Part model, mm, in its own coordinate system. Face numbers are marked on the shaded views. A direction names the side the tool comes from. Round coordinates to 2 decimals unless told otherwise and drop trailing zeros. Loops run counter-clockwise (first coordinate to the right, second up) from the corner with the lowest first, then second, coordinate; pieces in that order, holes last. Notation, with made-up numbers: M -5.5,7 L 52.5,7 A38 cw 52.5,46 Z; hole C 2.5,-27 d1. An arc over 180 degrees is marked long. Answer as CSV lines item,"result". Start each with the question number.
Item 1: Which spindle directions (+Z, -Z, +X, -X, +Y, -Y) get a long thin tool onto all of the face, cutting with end or side? Do the marked faces 4 and 5. Say none if no direction does.
Item 2: Band-saw the part on A-A (y = 0). Give the cut face in (x, z), and give its area (3 significant figures).
Item 3: Band-saw the part on B-B (z = 0). Give the cut face in (x, y), and give its area (3 significant figures).
Item 4: Wall check: line 1 (X direction, y = -0.5, z = 3.75); line 2 (X direction, y = 3.5, z = -1.75); line 3 (Y direction, x = 2, z = 4.5). Give the ranges that are in metal, low to high.
Item 5: Mould opens along Y. For the marked faces 1, 2 and 3 say: pulls with the +Y half, pulls with the -Y half, needs draft (parallel to the pull), parting line crosses it, or undercut.
Item 6: Drop flat-ended pins along their axis: pin 1 Ø5 at (x, y) = (6.5, 0.5) entering from +Z; pin 2 Ø4 at (x, y) = (13, -3.5) entering from +Z; pin 3 Ø0.7 at (x, z) = (1, 2) entering from +Y; pin 4 Ø6 at (y, z) = (-2, 3) entering from -X. Give the stop position or say it passes through.
Item 7: Band-saw the part on C-C (x = 4.5). Give the cut face in (y, z).
```python
from build123d import *

# Parameters (mm, degrees)
SKETCH1_R        = 6
BASEHEAD_DEPTH   = 3.6
BASEHEAD_DRAFT   = -3
SKETCH2_R        = 3
BASEBODY_DEPTH   = 14
HEADFILLET2_R    = 1.8
NOTCH_DEPTH      = 19.96325394
NOTCH_DEPTH_BACK = 19.96325394
SKETCH3_W        = 1.6
SKETCH3_H        = 1.4
HEADFILLET1_R    = 0.25


with BuildPart() as part:
    # Sketch1 → BaseHead (with draft: the straight prism first)
    with BuildSketch(Plane(origin=(3.6, 0, 0), x_dir=(0, 0, -1), z_dir=(1, 0, 0))):
        Circle(SKETCH1_R)
    extrude(amount=-BASEHEAD_DEPTH)
    # BaseHead: the draft: its side faces are tilted about the plane it starts from
    basehead_sides = [part.faces().sort_by_distance(p)[0] for p in [
        (1.8, 0, 6),
    ]]
    draft(basehead_sides, Plane(origin=(3.6, 0, 0), x_dir=(0, 0, -1), z_dir=(1, 0, 0)), BASEHEAD_DRAFT)

    # Sketch2 → BaseBody (add)
    with BuildSketch(Plane(origin=(3.6, 0, 0), x_dir=(0, 0, -1), z_dir=(1, 0, 0))):
        Circle(SKETCH2_R)
    extrude(amount=BASEBODY_DEPTH)

    # HeadFillet2
    headfillet2_edges = [part.edges().sort_by_distance(p)[0] for p in [
        (0, 0, 5.811331995),
    ]]
    fillet(headfillet2_edges, radius=HEADFILLET2_R)

    # Sketch3 → Notch (cut, two sides: drawn at the far end of the back side and taken through both)
    with BuildSketch(Plane(origin=(1.05, -1.05, 0), x_dir=(0, -1, 0), z_dir=(0, 0, 1)).offset(-NOTCH_DEPTH_BACK)):
        with Locations((-1.05, -0.35)):
            Rectangle(SKETCH3_W, SKETCH3_H)
    extrude(amount=NOTCH_DEPTH + NOTCH_DEPTH_BACK, mode=Mode.SUBTRACT)

    # HeadFillet1
    headfillet1_edges = [part.edges().sort_by_distance(p)[0] for p in [
        (3.6, 0, 3),
    ]]
    fillet(headfillet1_edges, radius=HEADFILLET1_R)


solid = part.part
```
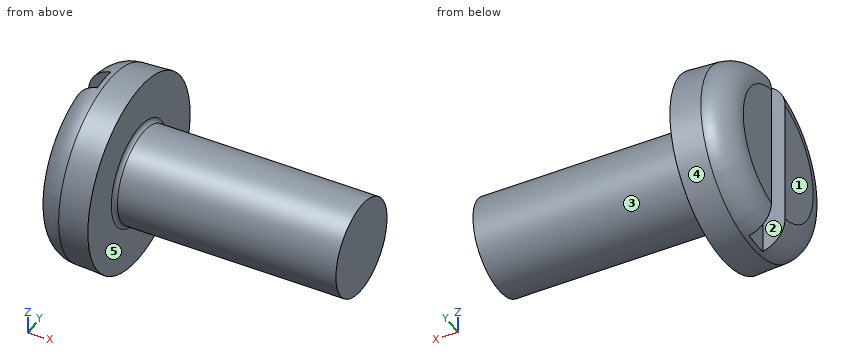
Answer block:
1,face 4,"-X"
1,face 5,"+X"
2,outline,"M 1.4,-5.86 A1.8 ccw 1.71,-5.9 L 3.6,-6 L 3.6,-3.25 A0.25 cw 3.85,-3 L 17.6,-3 L 17.6,3 L 3.85,3 A0.25 cw 3.6,3.25 L 3.6,6 L 1.71,5.9 A1.8 ccw 1.4,5.86 Z"
2,area,"110 mm^2"
3,outline,"M 0,-4.1 A1.8 ccw 1.71,-5.9 L 3.6,-6 L 3.6,-3.25 A0.25 cw 3.85,-3 L 17.6,-3 L 17.6,3 L 3.85,3 A0.25 cw 3.6,3.25 L 3.6,6 L 1.71,5.9 A1.8 ccw 0,4.1 L 0,0.8 L 1.4,0.8 L 1.4,-0.8 L 0,-0.8 Z"
3,area,"123 mm^2"
4,line 1,"x = 1.4 to 3.6"
4,line 2,"x = 0 to 3.6"
4,line 3,"y = -3.84 to 3.84"
5,face 1,"needs draft"
5,face 2,"undercut"
5,face 3,"parting line crosses it"
6,pin 1,"stops at z = 3"
6,pin 2,"stops at z = 2.6"
6,pin 3,"stops at y = 5.55"
6,pin 4,"stops at x = 0"
7,outline,"C 0,0 d6"
